Can you work these out from the model? Positions are in its coordinate system, mm. A direction names the side the tool comes from. Round coordinates to 2 decimals unless told otherwise and drop trailing zeros. Loops run counter-clockwise (first coordinate to the right, second up) from the corner with the lowest first, then second, coordinate; pieces in that order, holes last. Notation, with made-up numbers: (8.5, 87) -> (60.5, 87) arc R30 ccw to (60.5, 117) -> close; hole circle Ø3 at (-30.75, 30). An arc over 180 degrees is marked (long way). Answer as a JSON object with one key per item and string values.
Autodesk Inventor part; units mm, degrees
ref_plane "YZ Plane" through (0, 0, 0) normal (1, 0, 0) x (0, 1, 0)
ref_plane "XZ Plane" through (0, 0, 0) normal (0, 1, 0) x (-1, 0, 0)
ref_plane "XY Plane" through (0, 0, 0) normal (0, 0, 1) x (1, 0, 0)
ref_plane "작업 평면1" through (0, 0, 0) normal (0, 0, 1) x (1, 0, 0)
sketch "스케치1" plane through (0, 0, 0) normal (0, 0, 1) x (1, 0, 0)
  line L0 (42.4906, -94.9526) -> (42.4906, 93.0474)
  line L1 (42.4906, 93.0474) -> (-42.5094, 93.0474)
  line L2 (-42.5094, 93.0474) -> (-42.5094, -94.9526)
  line L3 (-42.5094, -94.9526) -> (42.4906, -94.9526)
  line L4 (0, 0) -> (0, 35)
  line L5 (0, 0) -> (25, 0)
  line L6 (0, 0) -> (0, -35)
  line L7 (0, 0) -> (-25, 0)
  line L8 (25, 35) -> (-25, 35)
  line L9 (-25, 35) -> (-25, -35)
  line L10 (-25, -35) -> (25, -35)
  line L11 (25, -35) -> (25, 35)
  line L12 (35, 45) -> (-35, 45)
  line L13 (-35, 45) -> (-35, -45)
  line L14 (-35, -45) -> (35, -45)
  line L15 (35, -45) -> (35, 45)
  line L16 (35, 45) -> (38, 45)
  line L17 (38, 45) -> (32, 45)
  line L18 (32, 45) -> (32, -45)
  line L19 (32, -45) -> (38, -45)
  line L20 (38, -45) -> (38, 45)
  line L21 (-35, 45) -> (-38, 45)
  line L22 (-38, 45) -> (-38, 42)
  line L23 (-38, 42) -> (-35, 42)
  line L24 (-35, 42) -> (-35, 45)
  line L25 (-38, 45) -> (-32, 45)
  line L26 (-32, 45) -> (-32, -45)
  line L27 (-32, -45) -> (-38, -45)
  line L28 (-38, -45) -> (-38, 45)
  circle A0 centre (7, -59) radius 1.25
  circle A1 centre (-1, 59) radius 1.25
  circle A2 centre (-1, -59) radius 1.25
  circle A3 centre (7, 59) radius 1.25
  dimension "d0" = 35
  dimension "d1" = 25
  dimension "d2" = 35
  dimension "d3" = 25
  dimension "d4" = 10
  dimension "d5" = 3
  dimension "d6" = 6
  dimension "d7" = 3
  dimension "d8" = 3
  dimension "d9" = 6
extrude "돌출1" add sketch "스케치1" along normal blind 35 contours L15 L14 L18 L12 | L16 L20 L19 L15
sketch "스케치2" plane through (38, -45, 0) normal (1, 0, 0) x (0, 0, -1)
  circle A0 centre (-27, 82) radius 1.25
  line L0 (-22, 77) -> (-32, 77)
  line L1 (-32, 77) -> (-32, 87)
  line L2 (-32, 87) -> (-22, 87)
  line L3 (-22, 87) -> (-22, 77)
  circle A1 centre (-27, 6.5) radius 1.25
  line L4 (-32, 3) -> (-32, 10)
  line L5 (-22, 10) -> (-32, 10)
  line L6 (-22, 3) -> (-22, 10)
  line L7 (-32, 3) -> (-22, 3)
  point P0 (0, 45)
extrude "돌출2" cut sketch "스케치2" against normal blind 35 contours A0 | A1
sketch "스케치3" plane through (38, -45, 0) normal (1, 0, 0) x (0, 0, -1)
  circle A0 centre (-27, 82) radius 1.25
  circle A1 centre (-27, 6.5) radius 1.25
  line L0 (0, 0) -> (0, 90)
  line L1 (0, 90) -> (-35, 90)
  line L2 (-35, 0) -> (-35, 90)
  line L3 (0, 0) -> (-35, 0)
  line L4 (0, 0) -> (-35, 0)
  line L5 (-35, 0) -> (-35, 90)
  line L6 (0, 0) -> (0, 90)
  line L7 (-27, 15) -> (-8, 15)
  line L8 (-8, 15) -> (-8, 18)
  line L9 (-8, 18) -> (-27, 18)
  line L10 (-27, 18) -> (-27, 15)
  line L11 (0, 90) -> (-35, 90)
  line L12 (-27, 75) -> (-8, 75)
  line L13 (-8, 75) -> (-8, 72)
  line L14 (-8, 72) -> (-27, 72)
  line L15 (-27, 72) -> (-27, 75)
  point P0 (0, 45)
  point P1 (-18.9095, 15)
  point P2 (-17.5, 0)
  point P3 (-8, 18.9545)
  point P4 (-18.9095, 75)
  point P5 (-17.5, 90)
  point P6 (-27, 64.4269)
  dimension "d14" = 15
  dimension "d15" = 8
  dimension "d16" = 8
  dimension "d17" = 3
  dimension "d18" = 15
  dimension "d19" = 8
  dimension "d20" = 3
extrude "돌출3" cut sketch "스케치3" against normal blind 35 contours L10 L9 L8 L7 | L12 L13 L14 L15
properties part number "60" material "아크릴, 선명"
Q1. If I drill on L1, parallel to Y at x = 35.15, z = 10.5, over which ranges is the centre line in solid material (lowest first)? Write a range as [from, to].
Determined:
{"L1": "[-45, -30], [-27, 27], [30, 45]"}
Q2. We'd pull the mould along Z, two halves only. Please class faces 3 (the flat face through (35, 1, 0)), 4 (the flat face through (35, -29, 8)), 5 (the flat face through (35, 1, 35)), 6 (the flat face through (38, -1, 17)): pulls with the +Z half, pulls with the -Z half, needs draft (parallel to the pull), parting line crosses it, or undercut.
Determined:
{"face 3": "pulls with the -Z half", "face 4": "undercut", "face 5": "pulls with the +Z half", "face 6": "needs draft"}
Q3. I want a section at B-B, the plane y = -38.5. Write out the boundary of the cut face in (x, z), then the cut area to 3 significant figures.
Determined:
{"outline": "(32, 0) -> (38, 0) -> (38, 25.75) -> (32, 25.75) -> close; (32, 28.25) -> (38, 28.25) -> (38, 35) -> (32, 35) -> close", "area": "195 mm²"}
Q4. I want a section at C-C, the plane x = 36.2. Write out the boundary of the cut face in (y, z).
Determined:
{"outline": "(-45, 0) -> (45, 0) -> (45, 35) -> (-45, 35) -> close; hole circle Ø2.5 at (-38.5, 27); hole (-30, 8) -> (-27, 8) -> (-27, 27) -> (-30, 27) -> close; hole (27, 8) -> (30, 8) -> (30, 27) -> (27, 27) -> close; hole circle Ø2.5 at (37, 27)"}
Q5. On a 3-axis mill with a long thin cutter (end or side, diameter ignored), from which of +Z, -Z, +X, -X, +Y, -Y can I reach the whole of each face in a straight line? I mean faces 1 (the flat face through (32, 1, 17)), 2 (the flat face through (35, -30, 18)). Say none if no direction works.
Determined:
{"face 1": "+Z, -Z, -X, +Y, -Y", "face 2": "+X, -X"}
Q6. I want a section at A-A, the plane z = 18. Write out the boundary of the cut face in (x, y).
Determined:
{"outline": "(32, -45) -> (38, -45) -> (38, -30) -> (32, -30) -> close; (32, -27) -> (38, -27) -> (38, 27) -> (32, 27) -> close; (32, 30) -> (38, 30) -> (38, 45) -> (32, 45) -> close"}
